Source: CAD feature listing. Evaluate the final solid. Frame: model axes, mm. A direction names the side the tool comes from. Round coordinates to 2 decimals unless told otherwise and drop trailing zeros. Write each loop counter-clockwise with the first axis right and the second up, starting at its lowest first coordinate (ties: lowest second). Pieces come first, ordered by that corner, then holes.
from build123d import *

# Parameters (mm, degrees)
SKETCH1_W           = 71.12
SKETCH1_H           = 106.68
BOSS_EXTRUDE1_DEPTH = 5.08
SKETCH3_W           = 25.908
SKETCH3_H           = 45.7962
SKETCH3_W_2         = 21.59
SKETCH3_H_2         = 41.4782
BOSS_EXTRUDE2_DEPTH = 27.305
SKETCH4_W           = 25.908
SKETCH4_H           = 54.1782
SKETCH4_W_2         = 21.59
SKETCH4_H_2         = 41.4782
BOSS_EXTRUDE3_DEPTH = 3.175
SKETCH5_R           = 2.04968221
CUT_EXTRUDE1_DEPTH  = 3.175
SKETCH7_W           = 15.748
SKETCH7_H           = 20.32
CUT_EXTRUDE3_DEPTH  = 45.7962
SKETCH8_R           = 10.16
BOSS_EXTRUDE4_DEPTH = 7.62
SKETCH9_R           = 8.255
CUT_EXTRUDE4_DEPTH  = 5.08
SKETCH10_W          = 20.32
SKETCH10_H          = 8.89
CUT_EXTRUDE5_DEPTH  = 6.08
SKETCH11_R          = 1.5875
CUT_EXTRUDE6_DEPTH  = 6.08
SKETCH15_R          = 2.921
CUT_EXTRUDE7_DEPTH  = 3.81
SKETCH16_R          = 2.921
CUT_EXTRUDE8_DEPTH  = 3.81
SKETCH17_R          = 1.5875
CUT_EXTRUDE9_DEPTH  = 36.56


with BuildPart() as part:
    # Sketch1 → Boss-Extrude1 (new body)
    with BuildSketch(Plane(origin=(56.401870569, 0, 2.613156724), x_dir=(1, 0, 0), z_dir=(0, 1, 0))):
        with Locations((-28.531301018, -3.803535099)):
            Rectangle(SKETCH1_W, SKETCH1_H)
    extrude(amount=BOSS_EXTRUDE1_DEPTH)

    # Sketch3 → Boss-Extrude2 (add)
    with BuildSketch(Plane(origin=(56.401870569, 5.08, 2.613156724), x_dir=(1, 0, 0), z_dir=(0, 1, 0))):
        with Locations((-28.531301018, 13.938364901)):
            Rectangle(SKETCH3_W, SKETCH3_H)
        with Locations((-28.531301018, 13.938364901)):
            Rectangle(SKETCH3_W_2, SKETCH3_H_2, mode=Mode.SUBTRACT)
    extrude(amount=BOSS_EXTRUDE2_DEPTH)

    # Sketch4 → Boss-Extrude3 (add)
    with BuildSketch(Plane(origin=(0, 32.385, 0), x_dir=(1, 0, 0), z_dir=(0, 1, 0))):
        with Locations((27.87056955, 11.325208176)):
            Rectangle(SKETCH4_W, SKETCH4_H)
        with Locations((27.87056955, 11.325208176)):
            Rectangle(SKETCH4_W_2, SKETCH4_H_2, mode=Mode.SUBTRACT)
    extrude(amount=BOSS_EXTRUDE3_DEPTH)

    # Sketch5 → Cut-Extrude1 (cut)
    with BuildSketch(Plane(origin=(0, 35.56, 0), x_dir=(1, 0, 0), z_dir=(0, 1, 0))):
        with Locations((22.19366955, 36.471208176)):
            Circle(SKETCH5_R)
        with Locations((33.54746955, 36.471208176)):
            Circle(SKETCH5_R)
        with Locations((22.19366955, -13.820791824)):
            Circle(SKETCH5_R)
        with Locations((33.54746955, -13.820791824)):
            Circle(SKETCH5_R)
    extrude(amount=-CUT_EXTRUDE1_DEPTH, mode=Mode.SUBTRACT)

    # Sketch7 → Cut-Extrude3 (cut)
    with BuildSketch(Plane(origin=(0, 0, -34.223308176), x_dir=(-1, 0, 0), z_dir=(0, 0, -1))):
        with Locations((-27.87056955, 15.24)):
            Rectangle(SKETCH7_W, SKETCH7_H)
    extrude(amount=-CUT_EXTRUDE3_DEPTH, mode=Mode.SUBTRACT)

    # Sketch8 → Boss-Extrude4 (add)
    with BuildSketch(Plane(origin=(0, 5.08, 0), x_dir=(1, 0, 0), z_dir=(0, 1, 0))):
        with Locations((27.87056955, -31.816691824)):
            Circle(SKETCH8_R)
    extrude(amount=BOSS_EXTRUDE4_DEPTH)

    # Sketch9 → Cut-Extrude4 (cut)
    with BuildSketch(Plane(origin=(0, 12.7, 0), x_dir=(1, 0, 0), z_dir=(0, 1, 0))):
        with Locations((27.87056955, -31.816691824)):
            Circle(SKETCH9_R)
    extrude(amount=-CUT_EXTRUDE4_DEPTH, mode=Mode.SUBTRACT)

    # Sketch10 → Cut-Extrude5 (cut, through all)
    with BuildSketch(Plane(origin=(0, 5.08, 0), x_dir=(1, 0, 0), z_dir=(0, 1, 0))):
        with Locations((27.87056955, -16.017891824)):
            Rectangle(SKETCH10_W, SKETCH10_H)
    extrude(amount=-CUT_EXTRUDE5_DEPTH, mode=Mode.SUBTRACT)

    # Sketch11 → Cut-Extrude6 (cut, through all)
    with BuildSketch(Plane(origin=(0, 5.08, 0), x_dir=(1, 0, 0), z_dir=(0, 1, 0))):
        with Locations((44.38056955, 39.303308176)):
            Circle(SKETCH11_R)
        with Locations((11.36056955, -52.136691824)):
            Circle(SKETCH11_R)
    extrude(amount=-CUT_EXTRUDE6_DEPTH, mode=Mode.SUBTRACT)

    # Sketch15 → Cut-Extrude7 (cut)
    with BuildSketch(Plane(origin=(0, 5.08, 0), x_dir=(1, 0, 0), z_dir=(0, 1, 0))):
        with Locations((11.36056955, -52.136691824)):
            Circle(SKETCH15_R)
        with Locations((44.38056955, 39.303308176)):
            Circle(SKETCH15_R)
    extrude(amount=-CUT_EXTRUDE7_DEPTH, mode=Mode.SUBTRACT)

    # Sketch16 → Cut-Extrude8 (cut)
    with BuildSketch(Plane.XZ):
        with Locations((-1.33943045, 53.406691824)):
            Circle(SKETCH16_R)
        with Locations((57.08056955, 53.406691824)):
            Circle(SKETCH16_R)
        with Locations((57.08056955, -40.573308176)):
            Circle(SKETCH16_R)
        with Locations((-1.33943045, -40.573308176)):
            Circle(SKETCH16_R)
    extrude(amount=-CUT_EXTRUDE8_DEPTH, mode=Mode.SUBTRACT)

    # Sketch17 → Cut-Extrude9 (cut, through all)
    with BuildSketch(Plane.XZ):
        with Locations((-1.33943045, 53.406691824)):
            Circle(SKETCH17_R)
        with Locations((57.08056955, 53.406691824)):
            Circle(SKETCH17_R)
        with Locations((57.08056955, -40.573308176)):
            Circle(SKETCH17_R)
        with Locations((-1.33943045, -40.573308176)):
            Circle(SKETCH17_R)
    extrude(amount=-CUT_EXTRUDE9_DEPTH, mode=Mode.SUBTRACT)


solid = part.part
1) Pull-direction query (X, two-part tool) for faces 4 (the face through (27, 5.08, 6)), 5 (the face through (37, 34, 15.764)), 6 (the face through (-7.689, 3, 7)), 7 (the face through (17.711, 3, 16)); classes: released by +X, released by -X, zero draft, split by the parting line, or undercut.
Taken from the geometry:
face 4: undercut
face 5: zero draft
face 6: released by -X
face 7: undercut
2) Section query D-D on x = 27.5. Return the cut outline in (y, z) (3 decimals).
Taken from the geometry:
outline: (0, -46.923) - (5.08, -46.923) - (5.08, 11.573) - (0, 11.573) - close; (0, 20.463) - (5.08, 20.463) - (5.08, 21.663) - (12.7, 21.663) - (12.7, 23.57) - (7.62, 23.57) - (7.62, 40.063) - (12.7, 40.063) - (12.7, 41.97) - (5.08, 41.97) - (5.08, 59.757) - (0, 59.757) - close; (25.4, -34.223) - (32.385, -34.223) - (32.385, -38.414) - (35.56, -38.414) - (35.56, -32.064) - (25.4, -32.064) - close; (25.4, 9.414) - (35.56, 9.414) - (35.56, 15.764) - (32.385, 15.764) - (32.385, 11.573) - (25.4, 11.573) - close
3) Material intervals for line 1 (X direction, y = 34, z = 4); line 2 (Z direction, x = 32, y = 34.5); line 3 (Z direction, x = 36.5, y = 1.5), sorted ascending.
Taken from the geometry:
line 1: x = 14.92 to 17.08, 38.67 to 40.82
line 2: z = -38.41 to -37.82, -35.13 to -32.06, 9.41 to 12.48, 15.16 to 15.76
line 3: z = -46.92 to 11.57, 20.46 to 59.76
4) Section query A-A on y = 10. Return the cut outline in (x, z) (3 decimals).
Taken from the geometry:
outline: (14.917, -34.223) - (19.997, -34.223) - (19.997, -32.064) - (17.076, -32.064) - (17.076, 9.414) - (19.997, 9.414) - (19.997, 11.573) - (14.917, 11.573) - close; circle Ø20.32 at (27.871, 31.817); (35.745, -34.223) - (40.825, -34.223) - (40.825, 11.573) - (35.745, 11.573) - (35.745, 9.414) - (38.666, 9.414) - (38.666, -32.064) - (35.745, -32.064) - close; hole circle Ø16.51 at (27.871, 31.817)
5) Section query B-B on y = 19.5. Return the cut outline in (x, z).
Taken from the geometry:
outline: (14.92, -34.22) - (20, -34.22) - (20, -32.06) - (17.08, -32.06) - (17.08, 9.41) - (20, 9.41) - (20, 11.57) - (14.92, 11.57) - close; (35.74, -34.22) - (40.82, -34.22) - (40.82, 11.57) - (35.74, 11.57) - (35.74, 9.41) - (38.67, 9.41) - (38.67, -32.06) - (35.74, -32.06) - close
6) Reachability of faces 1 (the face through (33.467, 33.995, -34.423)), 2 (the face through (40.825, 20, -11)), 3 (the face through (14.917, 20, -11)) from +Z, -Z, +X, -X, +Y, -Y: full face, straight path, thin tool, end or side. Return the list, or none.
Taken from the geometry:
face 1: +Y
face 2: +Z, -Z, +X, +Y
face 3: +Z, -Z, -X, +Y
7) Section query C-C on x = -1.5. Return the cut outline in (y, z).
Taken from the geometry:
outline: (0, -46.92) - (5.08, -46.92) - (5.08, -42.15) - (3.81, -42.15) - (3.81, -43.49) - (0, -43.49) - close; (0, -37.66) - (3.81, -37.66) - (3.81, -38.99) - (5.08, -38.99) - (5.08, 51.83) - (3.81, 51.83) - (3.81, 50.49) - (0, 50.49) - close; (0, 56.32) - (3.81, 56.32) - (3.81, 54.99) - (5.08, 54.99) - (5.08, 59.76) - (0, 59.76) - close
8) Contact query for flat-ended pins moving along their axis: P1, Ø5, axis at y = 13.5, z = -19, coming from the -X side; P2, Ø1.5, axis at y = 24, z = -17, coming from the +X side; P3, Ø1, axis at x = 29, y = 34.5, coming from the +Z side. Output: stop coordinate, or through.
Taken from the geometry:
P1: stops at x = 14.92
P2: stops at x = 40.82
P3: stops at z = 15.76
